from build123d import *

# Parameters (mm, degrees)
F0_W          = 300
F0_H          = 400
F1_DEPTH      = 300
F0_W_2        = 220
F0_H_2        = 75
F2_DEPTH      = 400
F3_DEPTH      = 300
F4_DEPTH      = 20
F6_DEPTH      = 220
F7_W          = 49.88788
F7_H          = 42.84564
F8_DEPTH      = 20
F9_DEPTH      = 50
F9_DEPTH_BACK = 10


with BuildPart() as f1:
    # F0 (on Top) → F1 (new body)
    with BuildSketch(Plane.XY):
        Rectangle(F0_W, F0_H)
        Polygon((170, 166.666694), (170, 220), (115.122088, 220), (110, 220), (-110, 220), (-115.122088, 220), (-170, 220), (-170, 166.666694), (-170, -166.666694), (-170, -220), (-115.122088, -220), (115.122088, -220), (170, -220), (170, -166.666694), align=None)
        Rectangle(F0_W, F0_H, mode=Mode.SUBTRACT)
    extrude(amount=F1_DEPTH)

    # F0 (on Top) → F2 (join)
    with BuildSketch(Plane.XY):
        with Locations((0, 257.5)):
            Rectangle(F0_W_2, F0_H_2)
    extrude(amount=F2_DEPTH)

    # F0 (on Top) → F3 (cut)
    with BuildSketch(Plane.XY):
        Rectangle(F0_W, F0_H)
    extrude(amount=F3_DEPTH, mode=Mode.SUBTRACT)

    # F0 (on Top) → F4 (join)
    with BuildSketch(Plane.XY):
        Rectangle(F0_W, F0_H)
    extrude(amount=F4_DEPTH)

    # F5 (on face) → F6 (cut, through all)
    with BuildSketch(Plane(origin=(-110, 0, 0), x_dir=(0, -1, 0), z_dir=(-1, 0, 0))):
        Polygon((-295, 400), (-295, 361.107111), (-280.523896, 361.107111), (-220, 315.353394), (-220, 400), align=None)
    extrude(amount=-F6_DEPTH, mode=Mode.SUBTRACT)

    # F7 (on face) → F8 (cut, through all)
    with BuildSketch(Plane.XZ.offset(220)):
        with Locations((0, 278.57718)):
            Rectangle(F7_W, F7_H)
    extrude(amount=-F8_DEPTH, mode=Mode.SUBTRACT)

    # F0 (on Top) → F9 (join, two sides)
    with BuildSketch(Plane.XY) as f9_sk:
        Polygon((-170, 220), (-115.122088, 220), (-115.122088, 236.666694), (-185.122088, 236.666694), (-185.122088, 166.666694), (-170, 166.666694), align=None)
        Polygon((-115.122088, -236.666694), (-115.122088, -220), (-170, -220), (-170, -166.666694), (-185.122088, -166.666694), (-185.122088, -236.666694), align=None)
        Polygon((185.122088, -166.666694), (170, -166.666694), (170, -220), (115.122088, -220), (115.122088, -236.666694), (185.122088, -236.666694), align=None)
        Polygon((115.122088, 220), (170, 220), (170, 166.666694), (185.122088, 166.666694), (185.122088, 236.666694), (115.122088, 236.666694), align=None)
    extrude(amount=F9_DEPTH)
    extrude(f9_sk.sketch, amount=-F9_DEPTH_BACK)


solid = f1.part
Could you check a few things on this model? Use its own coordinates, in mm. A direction names the side the tool comes from. Give positions to 0.01 mm unless a question says otherwise; leave off trailing zeros. Order: outer loops, then holes, each group sorted by start corner. A loop starts at its lowest first (then second) coordinate and runs counter-clockwise, first axis right, second up. Notation, with made-up numbers: M 87.5,-12 L 135.5,-12 A27 cw 135.5,17 Z; hole C -6,21 d6. An arc over 180 degrees is marked long. One line per question, with ' | ' between items.
1. If I drill on line 1 (X direction, y = 123, z = 22); line 2 (Y direction, x = -61, z = 230); line 3 (Y direction, x = 139, z = 81), over which ranges is the centre line in solid material (lowest first)?
Results:
line 1: -170 to -150, 150 to 170 | line 2: -220 to -200, 200 to 295 | line 3: -220 to -200, 200 to 220
2. I want a section at B-B (x = -141). List the corners of the cut face in (y, z) for me.
Results:
outline: M -236.67,-10 L -220,-10 L -220,0 L 220,0 L 220,-10 L 236.67,-10 L 236.67,50 L 220,50 L 220,300 L 200,300 L 200,20 L -200,20 L -200,300 L -220,300 L -220,50 L -236.67,50 Z
3. I want a section at D-D (z = 293.5). List the corners of the cut face in (x, y) for me, and give its area (3 significant figures).
Results:
outline: M -170,-220 L -24.94,-220 L -24.94,-200 L -150,-200 L -150,200 L 150,200 L 150,-200 L 24.94,-200 L 24.94,-220 L 170,-220 L 170,220 L 110,220 L 110,295 L -110,295 L -110,220 L -170,220 Z | area: 45,100 mm²
4. We'd pull the mould along X, two halves only. Please class faces 1 (the face through (185.122, -202, 20)), 2 (the face through (-185.122, -201, 20)), 3 (the face through (-150, -3, 158)): +X half, -X half, draft (parallel to the pull), parting line (faces both ways), or undercut.
Results:
face 1: +X half | face 2: -X half | face 3: undercut
5. I want a section at C-C (y = 5). List the corners of the cut face in (x, z) for me.
Results:
outline: M -170,0 L 170,0 L 170,300 L 150,300 L 150,20 L -150,20 L -150,300 L -170,300 Z
6. I'm going to push flat-ended pins straight in: pin 1 (8 mm diameter, centred on y = 20.5, z = 157.5, fed in from +X); pin 2 (1.5 mm diameter, centred on x = -74, y = 107, fed in from +Z); pin 3 (16.5 mm diameter, centred on x = -179.5, z = 20.5, fed in from +Y). Where does each tip first touch, or does it pass through?
Results:
pin 1: x = 170 | pin 2: z = 20 | pin 3: y = 236.67
7. For faces 4 (the face through (-152, 1, 300)), 5 (the face through (-177, -166.667, 20)), 6 (the face through (-150, 236.667, 20)), 7 (the face through (-115.122, -228, 20)), 8 (the face through (-2, 3, 20)), which set-ups out of +Z, -Z, +X, -X, +Y, -Y let a thin tool reach every point of the face, with its end or its side?
Results:
face 4: +Z, +X, -X, -Y | face 5: +Z, -Z, -X | face 6: +Z, -Z, -X, +Y | face 7: +Z, -Z, -Y | face 8: +Z
8. I want a section at A-A (z = 44). List the corners of the cut face in (x, y) for me.
Results:
outline: M -185.12,-236.67 L -115.12,-236.67 L -115.12,-220 L 115.12,-220 L 115.12,-236.67 L 185.12,-236.67 L 185.12,-166.67 L 170,-166.67 L 170,166.67 L 185.12,166.67 L 185.12,236.67 L 115.12,236.67 L 115.12,220 L 110,220 L 110,295 L -110,295 L -110,220 L -115.12,220 L -115.12,236.67 L -185.12,236.67 L -185.12,166.67 L -170,166.67 L -170,-166.67 L -185.12,-166.67 Z; hole M -150,-200 L 150,-200 L 150,200 L -150,200 Z
